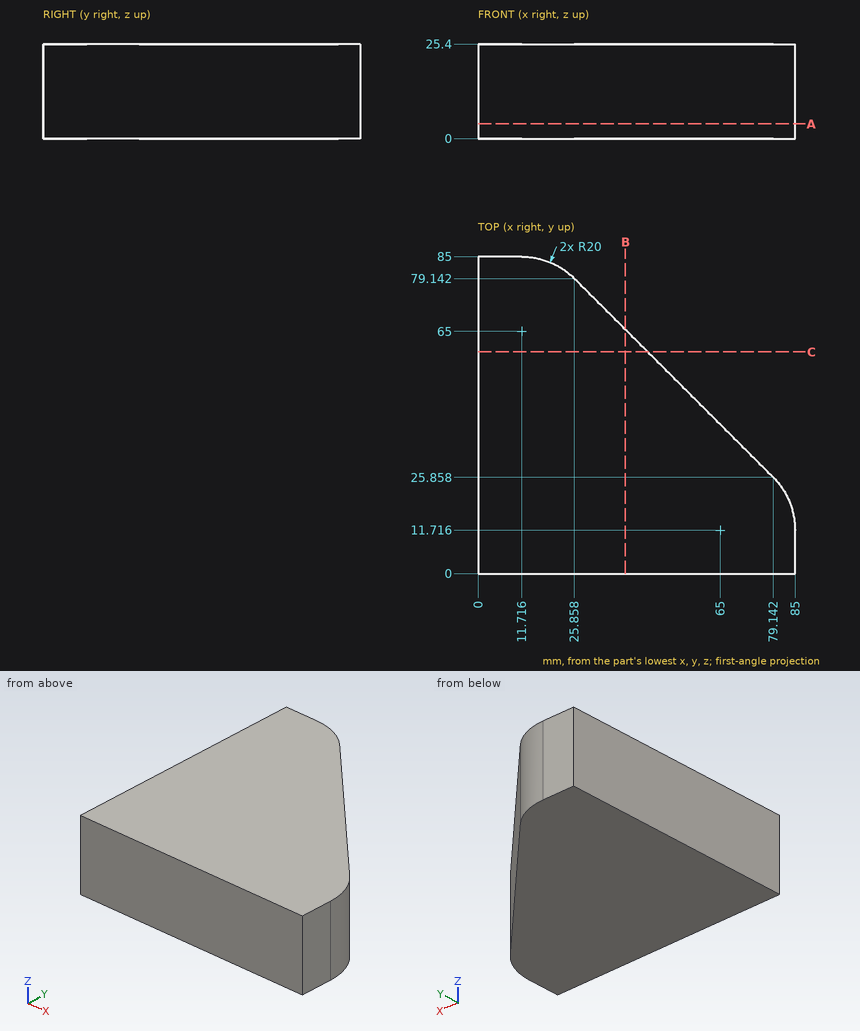
The drawing under review shows one solid part. Ordinate dimensions are in mm from its lowest x, y, z. Coordinates: 2 decimals unless noted, no trailing zeros. Loops run counter-clockwise (first coordinate to the right, second up) from the corner with the lowest first, then second, coordinate; pieces in that order, holes last. Notation, with made-up numbers: M 83.5,-19.5 L 113.5,-19.5 A22 ccw 113.5,7.5 Z; hole C -12.75,80.25 d2. An arc over 180 degrees is marked long. Use one line per item in the form item = value.
(1) Clearance check with a flat-ended pin moving along its axis: P1, Ø4, axis at y = 28, z = 3, coming from the +X side. State where the tip first meets the part, or that it passes through.
Return value:
P1 = 79
(2) For line 1 along Y through (x, z) = (12.5, 2) (1 decimal); line 2 along Y through (x, z) = (74, 11.75), list the stretches that pass through material, from the lowest coordinate up. Write a range as from..to.
Return value:
line_1 = 0..85
line_2 = 0..31
(3) Consider section C-C (y = 59.5). Write out the cut boundary in (x, z).
Return value:
outline = M 0,0 L 45.5,0 L 45.5,25.4 L 0,25.4 Z
(4) Consider section B-B (x = 39.5). Write out the cut boundary in (y, z).
Return value:
outline = M 0,0 L 65.5,0 L 65.5,25.4 L 0,25.4 Z
(5) Consider section A-A (z = 4). Write out the cut boundary in (x, y).
Return value:
outline = M 0,0 L 85,0 L 85,11.72 A20 ccw 79.14,25.86 L 25.86,79.14 A20 ccw 11.72,85 L 0,85 Z
